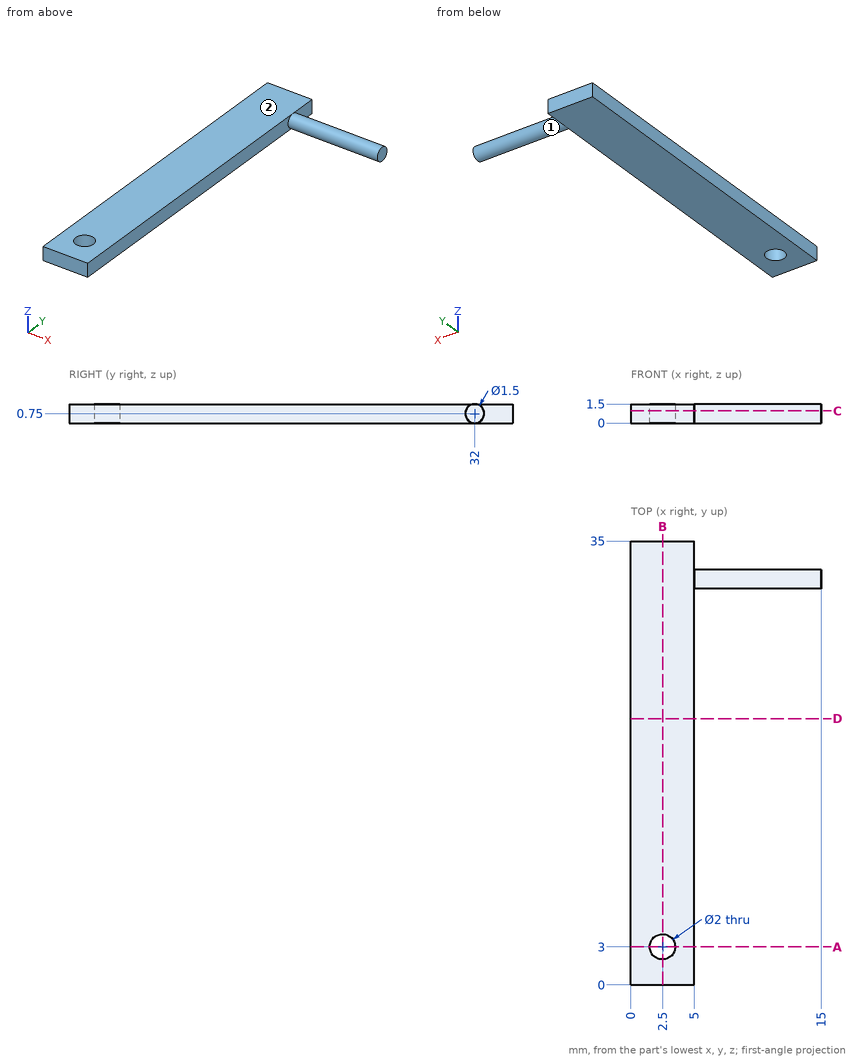
The drawing under review shows one solid part. Ordinate dimensions are in mm from its lowest x, y, z. A direction names the side the tool comes from. Coordinates: 2 decimals unless noted, no trailing zeros. Order: outer loops, then holes, each group sorted by start corner. A loop starts at its lowest first (then second) coordinate and runs counter-clockwise, first axis right, second up. Notation, with made-up numbers: (66, 21.25) - (125, 21.25) arc R34 cw to (125, 57.25) - close; hole circle Ø7 at (-0.75, -21.5). An arc over 180 degrees is marked (long way). Put each result on its own line as item: value.
1) Take a section at C-C, the plane z = 0.95. Give the boundary of the cut face in (x, y).
Response values:
outline: (0, 0) - (5, 0) - (5, 31.28) - (15, 31.28) - (15, 32.72) - (5, 32.72) - (5, 35) - (0, 35) - close; hole circle Ø2 at (2.5, 3)
2) Tool access review of the marked faces 1 and 2: name each direction out of +Z, -Z, +X, -X, +Y, -Y from which nothing blocks a thin tool from reaching the whole face with its end or side.
Response values:
face 1: +X
face 2: +Z, +X, -X, +Y, -Y
3) Take a section at D-D, the plane y = 21. Give the boundary of the cut face in (x, z).
Response values:
outline: (0, 0) - (5, 0) - (5, 1.5) - (0, 1.5) - close
4) Wall thickness on L1, parallel to Y at x = 2.5, z = 0.8; L2, parallel to Y at x = 3.25, z = 1.05; L3, parallel to X at y = 25.5, z = 0.55: over which ranges is each line inside the solid? List them lowest first. Write a range as from..to.
Response values:
L1: y = 0..2, 4..35
L2: y = 0..2.34, 3.66..35
L3: x = 0..5
5) Take a section at A-A, the plane y = 3. Give the boundary of the cut face in (x, z).
Response values:
outline: (0, 0) - (1.5, 0) - (1.5, 1.5) - (0, 1.5) - close; (3.5, 0) - (5, 0) - (5, 1.5) - (3.5, 1.5) - close
6) Take a section at B-B, the plane x = 2.5. Give the boundary of the cut face in (y, z), and give its area (3 significant figures).
Response values:
outline: (0, 0) - (2, 0) - (2, 1.5) - (0, 1.5) - close; (4, 0) - (35, 0) - (35, 1.5) - (4, 1.5) - close
area: 49.5 mm²
7) Insertion check: P1, Ø0.8, axis at y = 10.5, z = 1, coming from the +X side. The pin has a flat end and moves straight along its axis. Give the tip position at first contact, or say it passes through.
Response values:
P1: stops at x = 5
